The model under review builds one solid part; all positions refer to its coordinate system, in mm. Give positions to 0.01 mm unless a question says otherwise; leave off trailing zeros. Loops run counter-clockwise (first coordinate to the right, second up) from the corner with the lowest first, then second, coordinate; pieces in that order, holes last. Notation, with made-up numbers: (85, 0) -> (132, 0) arc R26 ccw to (132, 35) -> close; hole circle Ø4 at (71.5, 65.25). An arc over 180 degrees is marked (long way). Write each question's results on one line, items separated by ' | '. Start each with the question number.
Q1. We need section B-B (z = 79.5). Write out the cut boundary in (x, y).
Q2. Wall thickness on L1, parallel to X at y = 608, z = 323.85 (3 decimals); L2, parallel to X at y = 607, z = 431.8 (3 decimals); L3, parallel to X at y = 607.25, z = -215.9 (3 decimals): over which ranges is each line inside the solid? List them lowest first. Write a range as [from, to].
Q3. We need section A-A (x = -32). Write out the cut boundary in (y, z).
Q4. We need section C-C (y = 608). Give the number of separate pieces and of enclosed holes in the cut face, plus the area to 3 significant figures.
Q5. Insertion check: pin 1 Ø7.5 at (x, z) = (-171.45, -107.95) entering from +Y; pin 2 Ø5.5 at (x, z) = (57.15, 431.8) entering from -Y. Each pin has a flat end and moves straight along its axis. Give the tip position at first contact, or say it passes through.
from build123d import *

# Parameters (mm, degrees)
SKETCH1_W                   = 609.6
SKETCH1_H                   = 914.4
BOSS_EXTRUDE1_DEPTH         = 6.35
SKETCH2_W                   = 266.7
SKETCH2_H                   = 571.5
CUT_EXTRUDE1_DEPTH          = 7.35
FILLET1_R                   = 12.7
SKETCH3_R                   = 3.175
CUT_EXTRUDE2_DEPTH          = 7.35
F_1_4_0_25_DIAMETER_HOLE1_D = 6.35
LPATTERN1_COUNT             = 4
LPATTERN1_PITCH             = 114.3
F_1_4_0_25_DIAMETER_HOLE2_D = 6.35
LPATTERN2_COUNT             = 4
LPATTERN2_PITCH             = 114.3


with BuildPart() as part:
    # Sketch1 → Boss-Extrude1 (new body)
    with BuildSketch(Plane(origin=(0, 609.6, 0), x_dir=(1, 0, 0), z_dir=(0, 1, 0))):
        Rectangle(SKETCH1_W, SKETCH1_H)
    extrude(amount=-BOSS_EXTRUDE1_DEPTH)

    # Sketch2 → Cut-Extrude1 (cut, through all)
    with BuildSketch(Plane(origin=(0, 609.6, 0), x_dir=(1, 0, 0), z_dir=(0, 1, 0))):
        Rectangle(SKETCH2_W, SKETCH2_H)
    extrude(amount=-CUT_EXTRUDE1_DEPTH, mode=Mode.SUBTRACT)

    # Fillet1
    fillet1_edges = [part.edges().sort_by_distance(p)[0] for p in [
        (-133.35, 606.425, 285.75),
        (-133.35, 606.425, -285.75),
        (133.35, 606.425, -285.75),
        (133.35, 606.425, 285.75),
    ]]
    fillet(fillet1_edges, radius=FILLET1_R)

    # Sketch3 → Cut-Extrude2 (cut, through all)
    with BuildSketch(Plane(origin=(0, 609.6, 0), x_dir=(1, 0, 0), z_dir=(0, 1, 0))):
        with Locations((-171.45, 215.9)):
            Circle(SKETCH3_R)
        with Locations((-171.45, 107.95)):
            Circle(SKETCH3_R)
        with Locations((-171.45, 0)):
            Circle(SKETCH3_R)
        with Locations((-171.45, -107.95)):
            Circle(SKETCH3_R)
        with Locations((-171.45, -215.9)):
            Circle(SKETCH3_R)
        with Locations((-171.45, -323.85)):
            Circle(SKETCH3_R)
        with Locations((-85.725, -323.85)):
            Circle(SKETCH3_R)
        with Locations((0, -323.85)):
            Circle(SKETCH3_R)
        with Locations((85.725, -323.85)):
            Circle(SKETCH3_R)
        with Locations((171.45, -323.85)):
            Circle(SKETCH3_R)
        with Locations((171.45, -215.9)):
            Circle(SKETCH3_R)
        with Locations((171.45, -107.95)):
            Circle(SKETCH3_R)
        with Locations((171.45, 0)):
            Circle(SKETCH3_R)
        with Locations((171.45, 107.95)):
            Circle(SKETCH3_R)
        with Locations((171.45, 215.9)):
            Circle(SKETCH3_R)
        with Locations((171.45, 323.85)):
            Circle(SKETCH3_R)
        with Locations((85.725, 323.85)):
            Circle(SKETCH3_R)
        with Locations((0, 323.85)):
            Circle(SKETCH3_R)
        with Locations((-85.725, 323.85)):
            Circle(SKETCH3_R)
        with Locations((-171.45, 323.85)):
            Circle(SKETCH3_R)
    extrude(amount=-CUT_EXTRUDE2_DEPTH, mode=Mode.SUBTRACT)

    # 1/4 (0.25) Diameter Hole1 (through all)
    with Locations(Plane(origin=(0, 609.6, 0), x_dir=(1, 0, 0), z_dir=(0, 1, 0))):
        with Locations((171.45, -431.8)):
            f_1_4_0_25_diameter_hole1 = Hole(F_1_4_0_25_DIAMETER_HOLE1_D / 2)

    # LPattern1: 1/4 (0.25) Diameter Hole1 ×4
    with Locations(*[(-i * LPATTERN1_PITCH, 0, 0) for i in range(1, LPATTERN1_COUNT)]):
        add(f_1_4_0_25_diameter_hole1, mode=Mode.SUBTRACT)

    # 1/4 (0.25) Diameter Hole2 (through all)
    with Locations(Plane(origin=(0, 609.6, 0), x_dir=(1, 0, 0), z_dir=(0, 1, 0))):
        with Locations((-171.45, 431.8)):
            f_1_4_0_25_diameter_hole2 = Hole(F_1_4_0_25_DIAMETER_HOLE2_D / 2)

    # LPattern2: 1/4 (0.25) Diameter Hole2 ×4
    with Locations(*[(i * LPATTERN2_PITCH, 0, 0) for i in range(1, LPATTERN2_COUNT)]):
        add(f_1_4_0_25_diameter_hole2, mode=Mode.SUBTRACT)


solid = part.part
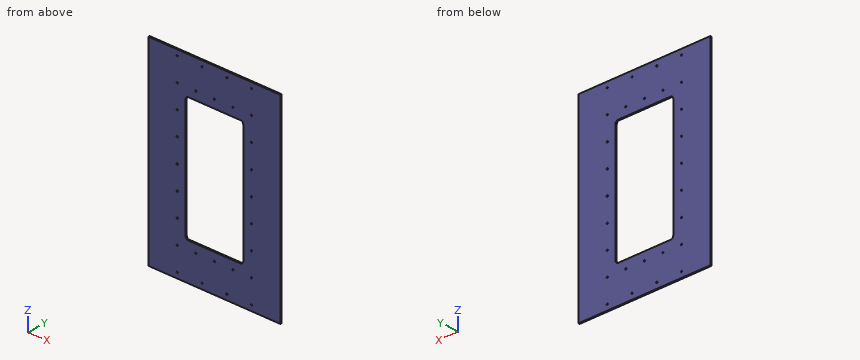
Output:
1) outline: (-304.8, 603.25) -> (-133.35, 603.25) -> (-133.35, 609.6) -> (-304.8, 609.6) -> close; (133.35, 603.25) -> (304.8, 603.25) -> (304.8, 609.6) -> (133.35, 609.6) -> close
2) L1: [-304.8, -174.625], [-168.275, -88.9], [-82.55, -3.175], [3.175, 82.55], [88.9, 168.275], [174.625, 304.8] | L2: [-304.8, -174.625], [-168.275, -60.325], [-53.975, 53.975], [60.325, 168.275], [174.625, 304.8] | L3: [-304.8, -174.625], [-168.275, -133.35], [133.35, 168.275], [174.625, 304.8]
3) outline: (603.25, -457.2) -> (609.6, -457.2) -> (609.6, -285.75) -> (603.25, -285.75) -> close; (603.25, 285.75) -> (609.6, 285.75) -> (609.6, 457.2) -> (603.25, 457.2) -> close
4) separate pieces: 1 | enclosed holes: 29 | area: 404,000 mm2
5) pin 1: y = 609.6 | pin 2: through
